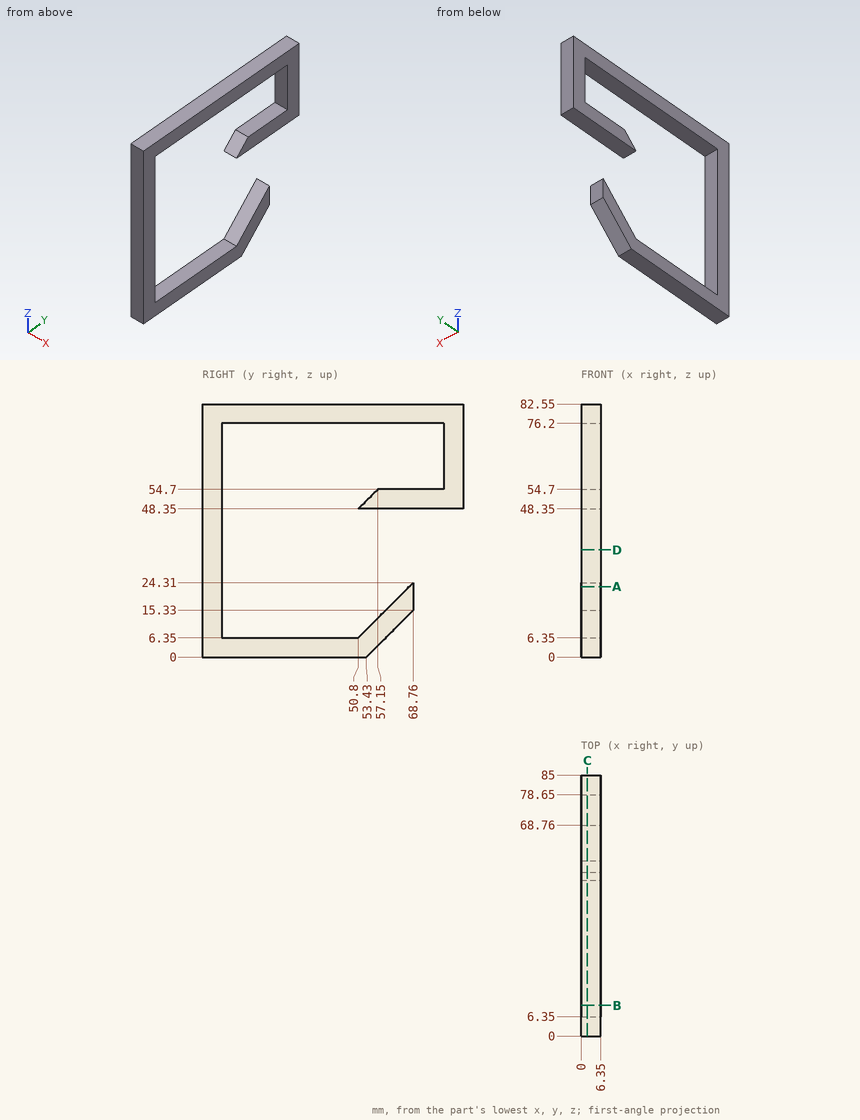
Source: three-view drawing plus pictorial views. Frame: mm from the lowest corner of the part. Coordinates: 2 decimals unless noted, no trailing zeros. Loops run counter-clockwise (first coordinate to the right, second up) from the corner with the lowest first, then second, coordinate; pieces in that order, holes last. Notation, with made-up numbers: (1, 21) -> (7, 21) arc R15 cw to (7, 32) -> close; hole circle Ø9 at (87.25, 50). An arc over 180 degrees is marked (long way). One line per item, written item: value.
(1) Cut plane C-C (x = 2). Output: boundary loops of the cut face in (y, z), then the cut area to 3 significant figures.
Answer below:
outline: (0, 0) -> (53.43, 0) -> (68.76, 15.33) -> (68.76, 24.31) -> (50.8, 6.35) -> (6.35, 6.35) -> (6.35, 76.2) -> (78.65, 76.2) -> (78.65, 54.7) -> (57.15, 54.7) -> (50.8, 48.35) -> (85, 48.35) -> (85, 82.55) -> (0, 82.55) -> close
area: 1,800 mm2
(2) Cut plane B-B (y = 10). Output: boundary loops of the cut face in (x, z).
Answer below:
outline: (0, 0) -> (6.35, 0) -> (6.35, 6.35) -> (0, 6.35) -> close; (0, 76.2) -> (6.35, 76.2) -> (6.35, 82.55) -> (0, 82.55) -> close
(3) Cut plane A-A (z = 23). Output: boundary loops of the cut face in (x, y).
Answer below:
outline: (0, 0) -> (6.35, 0) -> (6.35, 6.35) -> (0, 6.35) -> close; (0, 67.45) -> (6.35, 67.45) -> (6.35, 68.76) -> (0, 68.76) -> close
(4) Ray query, line 1 along Y through (x, z) = (2, 69); line 2 along Z through (x, y) = (1.75, 46.5); line 3 along Z through (x, y) = (1.5, 71). Return the intervals inside material, ascending.
Answer below:
line 1: y = 0 to 6.35, 78.65 to 85
line 2: z = 0 to 6.35, 76.2 to 82.55
line 3: z = 48.35 to 54.7, 76.2 to 82.55
(5) Cut plane D-D (z = 35). Output: boundary loops of the cut face in (x, y).
Answer below:
outline: (0, 0) -> (6.35, 0) -> (6.35, 6.35) -> (0, 6.35) -> close
(6) Pin query (flat end, axial travel): pin 1 Ø2 at (x, z) = (1.5, 22.5) entering from +Y. Return the tip coordinate at first contact, or that it passes through.
Answer below:
pin 1: stops at y = 68.76
